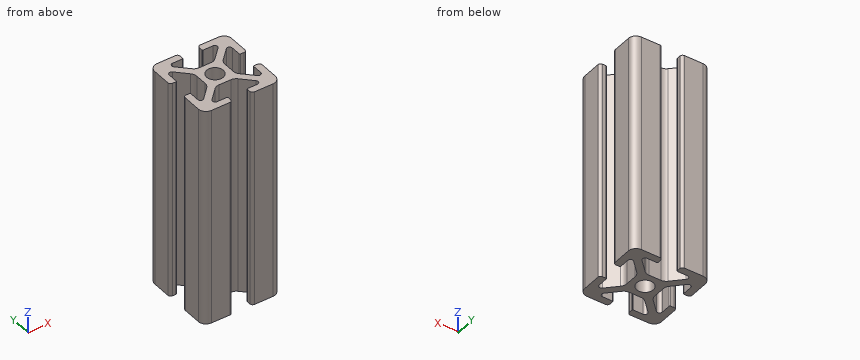
Autodesk Inventor part; units mm, degrees
ref_plane "YZ Plane" through (0, 0, 0) normal (1, 0, 0) x (0, 1, 0)
ref_plane "XZ Plane" through (0, 0, 0) normal (0, 1, 0) x (-1, 0, 0)
ref_plane "XY Plane" through (0, 0, 0) normal (0, 0, 1) x (1, 0, 0)
sketch "Sketch1" plane through (0, 0, 0) normal (0, 0, 1) x (1, 0, 0)
  circle A0 centre (0, 0) radius 2.15
  line L0 (-10, 10) -> (-2.5, 10)
  line L1 (-2.5, 10) -> (-2.5, 8.2)
  line L2 (-2.5, 8.2) -> (-6.9272, 8.2)
  line L3 (-6.9272, 8.2) -> (-2.3772, 3.65)
  line L4 (-2.3772, 3.65) -> (2.3772, 3.65)
  line L5 (2.3772, 3.65) -> (6.9272, 8.2)
  line L6 (6.9272, 8.2) -> (2.5, 8.2)
  line L7 (2.5, 8.2) -> (2.5, 10)
  line L8 (2.5, 10) -> (10, 10)
  line L9 (10, 10) -> (10, 2.5)
  line L10 (10, 2.5) -> (8.2, 2.5)
  line L11 (8.2, 2.5) -> (8.2, 6.9272)
  line L12 (8.2, 6.9272) -> (3.65, 2.3772)
  line L13 (3.65, 2.3772) -> (3.65, -2.3772)
  line L14 (3.65, -2.3772) -> (8.2, -6.9272)
  line L15 (8.2, -6.9272) -> (8.2, -2.5)
  line L16 (8.2, -2.5) -> (10, -2.5)
  line L17 (10, -2.5) -> (10, -10)
  line L18 (10, -10) -> (2.5, -10)
  line L19 (2.5, -10) -> (2.5, -8.2)
  line L20 (2.5, -8.2) -> (6.9272, -8.2)
  line L21 (6.9272, -8.2) -> (2.3772, -3.65)
  line L22 (2.3772, -3.65) -> (-2.3772, -3.65)
  line L23 (-2.3772, -3.65) -> (-6.9272, -8.2)
  line L24 (-6.9272, -8.2) -> (-2.5, -8.2)
  line L25 (-2.5, -8.2) -> (-2.5, -10)
  line L26 (-2.5, -10) -> (-10, -10)
  line L27 (-10, -10) -> (-10, -2.5)
  line L28 (-10, -2.5) -> (-8.2, -2.5)
  line L29 (-8.2, -2.5) -> (-8.2, -6.9272)
  line L30 (-8.2, -6.9272) -> (-3.65, -2.3772)
  line L31 (-3.65, -2.3772) -> (-3.65, 2.3772)
  line L32 (-3.65, 2.3772) -> (-8.2, 6.9272)
  line L33 (-8.2, 6.9272) -> (-8.2, 2.5)
  line L34 (-8.2, 2.5) -> (-10, 2.5)
  line L35 (-10, 2.5) -> (-10, 10)
  line L36 (0, 0) -> (-30.8654, 30.8654)
  line L37 (0, 0) -> (30.8654, 30.8654)
  line L38 (0, 0) -> (42.5392, 0)
  line L39 (0, 0) -> (0, 44.3419)
  dimension "d0" = 45
  dimension "d1" = 90
  dimension "Breite" = 20
  dimension "Tiefe_Schiene" = 6.35
  dimension "d2" = 1.8
  dimension "Durchmesser_Loch" = 4.3
  dimension "Wandstaerke" = 1.8
  dimension "d3" = 1.8
  dimension "Breite_Schiene" = 5
  dimension "d4" = 5
extrude "Extrusion1" add sketch "Sketch1" along normal mid plane 57 contours L38 L13 L14 L15 L16 L17 L18 L19 L20 L21 L22 L23 L24 L25 L26 L27 L28 L29 L30 L31 L32 L33 L34 L35 L36 A0 | A0 L37 L9 L10 L11 L12 L13 L38 | A0 L39 L4 L5 L6 L7 L8 L37 | L36 L0 L1 L2 L3 L4 L39 A0
fillet "Fillet1" radius 2 4 edges at (10, 10, 0) (-10, 10, 0) (10, -10, 0) (-10, -10, 0)
fillet "Fillet2" radius 0.2 8 edges at (-2.5, 8.2, 0) (2.5, 8.2, 0) (8.2, 2.5, 0) (8.2, -2.5, 0) (-2.5, -8.2, 0) (-8.2, -2.5, 0) (-8.2, 2.5, 0) (2.5, -8.2, 0)
fillet "Fillet3" radius 0.7 16 edges at (-2.5, 10, 0) (2.5, 10, 0) (10, 2.5, 0) (10, -2.5, 0) (2.5, -10, 0) (-2.5, -10, 0) (-10, -2.5, 0) (-10, 2.5, 0) (-6.9272, -8.2, 0) (-8.2, -6.9272, 0) (6.9272, -8.2, 0) (8.2, -6.9272, 0) (8.2, 6.9272, 0) (6.9272, 8.2, 0) (-6.9272, 8.2, 0) (-8.2, 6.9272, 0)
fillet "Fillet4" radius 2 8 edges at (-3.65, 2.3772, 0) (-2.3772, 3.65, 0) (2.3772, 3.65, 0) (3.65, 2.3772, 0) (3.65, -2.3772, 0) (2.3772, -3.65, 0) (-2.3772, -3.65, 0) (-3.65, -2.3772, 0)
equation "\"d2\" = Wandstaerke"
equation "\"d3\" = Wandstaerke"
equation "\"d4\" = Breite_Schiene"
properties part number "ITEM_20x20_77mm"
Verification items for the finished model (mm, model axes). Give positions to 0.01 mm unless a question says otherwise; leave off trailing zeros. Order: outer loops, then holes, each group sorted by start corner. A loop starts at its lowest first (then second) coordinate and runs counter-clockwise, first axis right, second up. Notation, with made-up numbers: M 87.25,4 L 143.25,4 A27 cw 143.25,34 Z; hole C -24,11 d8. An arc over 180 degrees is marked long. Answer as a JSON object with one key per item and string values. Group by question number.
1) Cross-section at A-A (y = 0). Enter the section's corners in (x, z), then the cut area to 3 significant figures.
2) Scan lines: line 1 along X through (y, z) = (0, 7); line 2 along Y through (x, z) = (5.5, 18.5). Record each from-to range of solid material in increasing order. Write a range as [from, to].
3) Depth check by flat-ended pin: pin 1 Ø0.5 at (x, z) = (-8.5, -10) entering from +Y; pin 2 Ø0.5 at (y, z) = (9, -9.5) entering from +X; pin 3 Ø0.5 at (y, z) = (-9, 5) entering from -X; pin 4 Ø4 at (x, y) = (0, 0) entering from +Z. Enter the tip coordinate at first touch or a pass-through.
Result sheet:
{
 "1": {"outline": "M -3.65,-28.5 L -2.15,-28.5 L -2.15,28.5 L -3.65,28.5 Z; M 2.15,-28.5 L 3.65,-28.5 L 3.65,28.5 L 2.15,28.5 Z", "area": "171 mm2"},
 "2": {"line 1": "x = [-3.65, -2.15], [2.15, 3.65]", "line 2": "y = [-10, -8.15], [-6.77, -4.23], [4.23, 6.77], [8.15, 10]"},
 "3": {"pin 1": "stops at y = 9.98", "pin 2": "stops at x = 9.85", "pin 3": "stops at x = -9.85", "pin 4": "passes through"}
}
